```python
from build123d import *

# Parameters (mm, degrees)
F1_DEPTH      = 20
F1_DEPTH_BACK = 20
F2_R          = 2
F3_DEPTH      = 25.4
F5_DEPTH      = 50.8
F7_DEPTH      = 2
F7_DEPTH_BACK = 2
F8_SIZE       = 2.54
F9_R          = 5.08
F10_T1_DEPTH  = 15.875
F11_T1_DEPTH  = 18.9511481059


# Not quite as in the source:
# - a fillet or chamfer that OpenCascade refuses, or shapes differently, is made with other operations: its cross-section is extruded or revolved along the edge and cut away or added


with BuildPart() as f1:
    # F0 (on Front) → F1 (new body, two sides)
    with BuildSketch(Plane.XZ) as f1_sk:
        with BuildLine():
            Line((0, 3.175), (0, 0))
            ThreePointArc((0, 0), (52.3634414453, 6.4462342186), (101.6, 25.4))
            Line((101.6, 25.4), (100.1058823529, 28.2014705882))
            ThreePointArc((100.1058823529, 28.2014705882), (51.5933908359, 9.5264366566), (0, 3.175))
        make_face()
    extrude(amount=F1_DEPTH)
    extrude(f1_sk.sketch, amount=-F1_DEPTH_BACK)

    # F2 (on Top) → F3 (cut)
    with BuildSketch(Plane.XY):
        with Locations((6, 14)):
            Circle(F2_R)
        with Locations((6, -14)):
            Circle(F2_R)
    extrude(amount=F3_DEPTH, mode=Mode.SUBTRACT)

    # F4 (on Top) → F5 (cut)
    with BuildSketch(Plane.XY):
        Polygon((0.5, 20), (101.6, 8), (101.6, 20), align=None)
        Polygon((101.6, -8), (0.5, -20), (101.6, -20), align=None)
    extrude(amount=F5_DEPTH, mode=Mode.SUBTRACT)

    # F6 (on Front) → F7 (join, two sides)
    with BuildSketch(Plane.XZ) as f7_sk:
        Polygon((0, 6), (0, 0), (37, 6), align=None)
    extrude(amount=F7_DEPTH)
    extrude(f7_sk.sketch, amount=-F7_DEPTH_BACK)

    # F8
    f8_edges = [f1.edges().sort_by_distance(p)[0] for p in [
        (17.334188, -2, 3.882426),
        (17.334188, 2, 3.882426),
    ]]
    chamfer(f8_edges, length=F8_SIZE)

    # F9
    f9_edges = [f1.edges().sort_by_distance(p)[0] for p in [
        (100.852941, -8.088672, 26.800735),
        (100.852941, 8.088672, 26.800735),
    ]]
    fillet(f9_edges, radius=F9_R)

    # F10: fillet of radius 2.54 on 2 edges, made by hand

    # F10_s2 → F10_t1 (cut)
    with BuildSketch(Plane.XY.offset(-6.35)):
        with BuildLine():
            ThreePointArc((0, -17.46), (0.7439487758, -19.2560512242), (2.54, -20))
            Line((2.54, -20), (0, -20))
            Line((0, -20), (0, -17.46))
        make_face()
        with BuildLine():
            ThreePointArc((2.54, 20), (0.7439487758, 19.2560512242), (0, 17.46))
            Line((0, 17.46), (0, 20))
            Line((0, 20), (2.54, 20))
        make_face()
    extrude(amount=F10_T1_DEPTH, mode=Mode.SUBTRACT)

    # F11: fillet of radius 2.54 on 2 edges, made by hand

    # F11_s2 → F11_t1 (cut)
    with BuildSketch(Plane.XY.offset(-7.8813228745)):
        with BuildLine():
            ThreePointArc((0, -17.2000338729), (0.8531139151, -19.0989849877), (2.8393821549, -19.7223285276))
            Line((2.8393821549, -19.7223285276), (2.8693203704, -19.9745579931))
            Line((2.8693203704, -19.9745579931), (1.7309730402, -20.1096734032))
            Line((1.7309730402, -20.1096734032), (1.6171383071, -20.0971883315))
            ThreePointArc((1.6171383071, -20.0971883315), (-0.254, -17.46), (-0.254, -17.2000338729))
            Line((-0.254, -17.2000338729), (0, -17.2000338729))
        make_face()
        with BuildLine():
            ThreePointArc((0, 17.2000338729), (0.8531139151, 19.0989849877), (2.8393821549, 19.7223285276))
            Line((2.8393821549, 19.7223285276), (2.8693203704, 19.9745579931))
            Line((2.8693203704, 19.9745579931), (1.7309730402, 20.1096734032))
            Line((1.7309730402, 20.1096734032), (1.6171383071, 20.0971883315))
            ThreePointArc((1.6171383071, 20.0971883315), (-0.254, 17.46), (-0.254, 17.2000338729))
            Line((-0.254, 17.2000338729), (0, 17.2000338729))
        make_face()
    extrude(amount=F11_T1_DEPTH, mode=Mode.SUBTRACT)


solid = f1.part
```
Geometry: final body of the model. Coordinates: model frame, mm. A direction names the side the tool comes from. Round coordinates to 2 decimals unless told otherwise and drop trailing zeros. Write each loop counter-clockwise with the first axis right and the second up, starting at its lowest first coordinate (ties: lowest second). Pieces come first, ordered by that corner, then holes.
Item 1: Section query B-B (y = 0.5). Return loops of the section in (x, z) (3 decimals).
Item 2: Section query C-C (x = 6). Give the number of separate pieces and of enclosed holes in the cut face, plus the area to 3 significant figures.
Item 3: Pin query (flat end, axial travel): P1, Ø6, axis at y = -5, z = 24.5, coming from the -X side; P2, Ø4.5, axis at x = 14, y = -1.5, coming from the +Z side; P3, Ø12, axis at x = 13.5, z = 10, coming from the -Y side; P4, Ø2.5, axis at x = 6, y = 14, coming from the +Z side. Return the tip coordinate at first contact, or that it passes through.
Item 4: Set-up query: faces 5 (the face through (21, 0, 6)), 6 (the face through (99.73, 6.872, 26.205)), 7 (the face through (52.301, -0.277, 9.705)). Return all of +Z, -Z, +X, -X, +Y, -Y with unobstructed straight access to the full face (end or side cutting, diameter ignored); none if empty.
Item 5: Material intervals for L1, parallel to Y at x = 6, z = 1.8; L2, parallel to X at y = -6, z = 22.75; L3, parallel to Z at x = 33, y = 7, sorted ascending.
Item 6: Section query A-A (y = -14). Return loops of the section in (x, z) (3 decimals), plus the area to 3 significant figures.
Item 7: Section query D-D (z = 17.5). Return loops of the section in (x, y).
Item 8: Mould query, pull axis X, two halves, no side actions, for faces 1 (the face through (99.69, -6.95, 26.12)), 2 (the face through (6, 16, 2)), 3 (the face through (6, -12, 2)), 4 (the face through (13.165, 3.252, 4.873)). Classes: +X half, -X half, draft (parallel to the pull), parting line (faces both ways), or undercut.
Completed:
1. outline: (0, 0) arc R215.9 ccw to (101.6, 25.4) - (100.106, 28.201) arc R212.725 cw to (34.553, 6) - (0, 6) - close
2. separate pieces: 3
2. enclosed holes: 0
2. area: 115 mm2
3. P1: stops at x = 86.37
3. P2: stops at z = 6
3. P3: stops at y = -4.16
3. P4: passes through
4. face 5: +Z, -X, +Y, -Y
4. face 6: +Z, +X, +Y
4. face 7: +Z, -X
5. L1: y = -19.35 to -16, -12 to 12, 16 to 19.35
5. L2: x = 89.13 to 96.47
5. L3: z = 2.54 to 5.75
6. outline: (0, 0) arc R215.9 ccw to (4, 0.037) - (4, 3.213) arc R212.725 cw to (0, 3.175) - close; (8, 0.148) arc R215.9 ccw to (51.05, 6.122) - (51.05, 9.391) arc R212.725 cw to (8, 3.325) - close
6. area: 151 mm2
7. outline: (76.74, -10.95) - (85.15, -9.95) - (85.15, 9.95) - (76.74, 10.95) - close
8. face 1: +X half
8. face 2: undercut
8. face 3: undercut
8. face 4: -X half
